```python
from build123d import *

# Parameters (mm, degrees)
SKETCH1_W           = 12.7
SKETCH1_H           = 50.038
SKETCH1_R           = 4.191
SKETCH1_R_2         = 2.286
SKETCH1_H_2         = 2.54
BOSS_EXTRUDE1_DEPTH = 1.905
BOSS_EXTRUDE3_START = 1.905
SKETCH1_3_W         = 7.62
SKETCH1_3_H         = 50.038
SKETCH1_3_W_2       = 12.7
SKETCH1_3_R         = 4.191
SKETCH1_3_H_2       = 2.54
BOSS_EXTRUDE3_DEPTH = 3.175
BOSS_EXTRUDE4_START = 5.08
SKETCH1_4_W         = 12.7
SKETCH1_4_H         = 2.54
BOSS_EXTRUDE4_DEPTH = 5.08
FILLET1_R           = 2.54


with BuildPart() as part:
    # Sketch1 → Boss-Extrude1 (new body)
    with BuildSketch(Plane(origin=(0, 0, 0), x_dir=(1, 0, 0), z_dir=(0, 1, 0))):
        with Locations((6.35, 25.019)):
            Rectangle(SKETCH1_W, SKETCH1_H)
        with Locations((6.35, 7.62)):
            Circle(SKETCH1_R, mode=Mode.SUBTRACT)
        with Locations((26.67, 25.019)):
            Rectangle(SKETCH1_W, SKETCH1_H)
        with Locations((26.67, 42.418)):
            Circle(SKETCH1_R, mode=Mode.SUBTRACT)
        with Locations((6.35, 7.62)):
            Circle(SKETCH1_R)
        with Locations((6.35, 7.62)):
            Circle(SKETCH1_R_2, mode=Mode.SUBTRACT)
        with Locations((26.67, 42.418)):
            Circle(SKETCH1_R)
        with Locations((26.67, 42.418)):
            Circle(SKETCH1_R_2, mode=Mode.SUBTRACT)
        Polygon((12.7, 0), (0, 0), (0, 50.038), (12.7, 50.038), (12.7, 52.578), (-2.54, 52.578), (-2.54, -2.54), (12.7, -2.54), align=None)
        with Locations((26.67, 51.308)):
            Rectangle(SKETCH1_W, SKETCH1_H_2)
        with Locations((26.67, -1.27)):
            Rectangle(SKETCH1_W, SKETCH1_H_2)
    extrude(amount=BOSS_EXTRUDE1_DEPTH)

    # Sketch1_3 → Boss-Extrude3 (add)
    with BuildSketch(Plane(origin=(0, 0, 0), x_dir=(1, 0, 0), z_dir=(0, 1, 0)).offset(BOSS_EXTRUDE3_START)):
        with Locations((16.51, 25.019)):
            Rectangle(SKETCH1_3_W, SKETCH1_3_H)
        with Locations((6.35, 25.019)):
            Rectangle(SKETCH1_3_W_2, SKETCH1_3_H)
        with Locations((6.35, 7.62)):
            Circle(SKETCH1_3_R, mode=Mode.SUBTRACT)
        with Locations((26.67, 25.019)):
            Rectangle(SKETCH1_3_W_2, SKETCH1_3_H)
        with Locations((26.67, 42.418)):
            Circle(SKETCH1_3_R, mode=Mode.SUBTRACT)
        Polygon((12.7, 0), (0, 0), (0, 50.038), (12.7, 50.038), (12.7, 52.578), (-2.54, 52.578), (-2.54, -2.54), (12.7, -2.54), align=None)
        with Locations((26.67, -1.27)):
            Rectangle(SKETCH1_3_W_2, SKETCH1_3_H_2)
        with Locations((26.67, 51.308)):
            Rectangle(SKETCH1_3_W_2, SKETCH1_3_H_2)
    extrude(amount=BOSS_EXTRUDE3_DEPTH)

    # Sketch1_4 → Boss-Extrude4 (add)
    with BuildSketch(Plane(origin=(0, 0, 0), x_dir=(1, 0, 0), z_dir=(0, 1, 0)).offset(BOSS_EXTRUDE4_START)):
        Polygon((12.7, 0), (0, 0), (0, 50.038), (12.7, 50.038), (12.7, 52.578), (-2.54, 52.578), (-2.54, -2.54), (12.7, -2.54), align=None)
        with Locations((26.67, -1.27)):
            Rectangle(SKETCH1_4_W, SKETCH1_4_H)
        with Locations((26.67, 51.308)):
            Rectangle(SKETCH1_4_W, SKETCH1_4_H)
    extrude(amount=BOSS_EXTRUDE4_DEPTH)

    # Fillet1
    fillet1_edges = [part.edges().sort_by_distance(p)[0] for p in [
        (0, 7.62, -50.038),
        (0, 7.62, 0),
        (-2.54, 5.08, -52.578),
        (-2.54, 5.08, 2.54),
        (16.51, 1.905, -50.038),
        (16.51, 1.905, 0),
    ]]
    fillet(fillet1_edges, radius=FILLET1_R)


solid = part.part
```
Geometry: final body of the model. Coordinates: model frame, mm. A direction names the side the tool comes from. Round coordinates to 2 decimals unless told otherwise and drop trailing zeros. Write each loop counter-clockwise with the first axis right and the second up, starting at its lowest first coordinate (ties: lowest second). Pieces come first, ordered by that corner, then holes. Notation, with made-up numbers: (17, 60.5) -> (32, 60.5) arc R16 cw to (32, 84.5) -> close; hole circle Ø8 at (6, 32.25). An arc over 180 degrees is marked (long way). Return JSON: item names as keys, results as strings.
Q1. Section B-B on z = -7.62. Return the cut outline in (x, y) (3 decimals).
From the geometry:
{"outline": "(-2.54, 0) -> (4.064, 0) -> (4.064, 1.905) -> (2.159, 1.905) -> (2.159, 5.08) -> (0, 5.08) -> (0, 10.16) -> (-2.54, 10.16) -> close; (8.636, 0) -> (12.7, 0) -> (12.7, 1.905) -> (20.32, 1.905) -> (20.32, 0) -> (33.02, 0) -> (33.02, 5.08) -> (10.541, 5.08) -> (10.541, 1.905) -> (8.636, 1.905) -> close"}
Q2. Section D-D on x = 21. Return the cut outline in (y, z), and give its area (3 significant figures).
From the geometry:
{"outline": "(0, -52.58) -> (10.16, -52.58) -> (10.16, -50.04) -> (5.08, -50.04) -> (5.08, 0) -> (10.16, 0) -> (10.16, 2.54) -> (0, 2.54) -> close", "area": "306 mm2"}
Q3. First-contact query: pin 1 Ø9.5 at (x, z) = (26.67, -42.418) entering from +Y; pin 2 Ø1 at (x, y) = (19, 5) entering from -Z; pin 3 Ø2 at (x, z) = (28.5, -35.5) entering from -Y; pin 4 Ø2.5 at (x, z) = (18, -27) entering from -Y (3 decimals). Flat tips, straight axial feed; report the tip coordinate or a pass-through.
From the geometry:
{"pin 1": "y = 5.08", "pin 2": "z = -50.04", "pin 3": "y = 0", "pin 4": "y = 1.905"}
Q4. Mould query, pull axis Z, two halves, no side actions, for faces 1 (the flat face through (5, 0, -25)), 2 (the flat face through (8.2, 1.905, -5.8)), 3 (the cylindrical face through (-1.82, 5.15, -51.81)). Classes: +Z half, -Z half, draft (parallel to the pull), parting line (faces both ways), or undercut.
From the geometry:
{"face 1": "draft", "face 2": "undercut", "face 3": "-Z half"}
Q5. Ray query, line 1 (Z direction, x = 26.67, y = 3.9); line 2 (X direction, y = 1, z = -1); line 3 (Y direction, x = 15, z = -9.5) (3 decimals). Return the intervals inside material, ascending.
From the geometry:
{"line 1": "-52.58 to -46.61, -38.23 to 2.54", "line 2": "-2.54 to 12.7, 20.32 to 33.02", "line 3": "1.905 to 5.08"}
Q6. Section A-A on y = 7. Return the cut outline in (x, z), and give its area (3 significant figures).
From the geometry:
{"outline": "(-2.54, -50.04) arc R2.54 ccw to (0, -52.58) -> (12.7, -52.58) -> (12.7, -50.04) -> (2.54, -50.04) arc R2.54 cw to (0, -47.5) -> (0, -2.54) arc R2.54 cw to (2.54, 0) -> (12.7, 0) -> (12.7, 2.54) -> (0, 2.54) arc R2.54 ccw to (-2.54, 0) -> close; (20.32, -52.58) -> (33.02, -52.58) -> (33.02, -50.04) -> (20.32, -50.04) -> close; (20.32, 0) -> (33.02, 0) -> (33.02, 2.54) -> (20.32, 2.54) -> close", "area": "269 mm2"}
Q7. Set-up query: faces 4 (the cylindrical face through (5.44, 3.47, -3.53)), 5 (the flat face through (8, 8, 0)), 6 (the cylindrical face through (16.563, 2.629, -0.764)), 7 (the flat face through (-1, 10.16, -21)), 8 (the flat face through (16, 1.905, -25)). Return all of +Z, -Z, +X, -X, +Y, -Y with unobstructed straight access to the full face (end or side cutting, diameter ignored); none if empty.
From the geometry:
{"face 4": "+Y", "face 5": "+X, +Y", "face 6": "+Z, -Y", "face 7": "+Z, -Z, +X, -X, +Y", "face 8": "+Z, -Z, -Y"}
Q8. Section C-C on x = 6.35. Return the cut outline in (y, z) (3 decimals).
From the geometry:
{"outline": "(0, -52.578) -> (10.16, -52.578) -> (10.16, -50.038) -> (5.08, -50.038) -> (5.08, -11.811) -> (1.905, -11.811) -> (1.905, -9.906) -> (0, -9.906) -> close; (0, -5.334) -> (1.905, -5.334) -> (1.905, -3.429) -> (5.08, -3.429) -> (5.08, 0) -> (10.16, 0) -> (10.16, 2.54) -> (0, 2.54) -> close"}
